```python
from build123d import *

# Parameters (mm, degrees)
F0_R      = 56.35625
F1_DEPTH  = 2120.9
F2_R      = 50.8
F3_DEPTH  = 368.3
F4_R      = 11.1125
F5_DEPTH  = 34.925
F6_W      = 25.4
F6_H      = 25.4
F7_DEPTH  = 355.6
F8_R      = 12.699
F11_DEPTH = 13.97


# Not quite as in the source:
# - a fillet or chamfer is up to 0.001 mm smaller than in the source, because OpenCascade refuses the exact size


with BuildPart() as f1:
    # F0 (on Front) → F1 (new body)
    with BuildSketch(Plane.XZ):
        Circle(F0_R)
    extrude(amount=-F1_DEPTH)

    # F2 (on face) → F3 (join)
    with BuildSketch(Plane(origin=(0, 2120.9, 0), x_dir=(-1, 0, 0), z_dir=(0, 1, 0))):
        Circle(F2_R)
    extrude(amount=F3_DEPTH)

    # F4 (on face) → F5 (cut)
    with BuildSketch(Plane(origin=(0, 2489.2, 0), x_dir=(-1, 0, 0), z_dir=(0, 1, 0))):
        Circle(F4_R)
    extrude(amount=-F5_DEPTH, mode=Mode.SUBTRACT)

    # F6 (on face) → F7 (cut)
    with BuildSketch(Plane(origin=(0, 2489.2, 0), x_dir=(-1, 0, 0), z_dir=(0, 1, 0))):
        with Locations((0, 49.53)):
            Rectangle(F6_W, F6_H)
    extrude(amount=-F7_DEPTH, mode=Mode.SUBTRACT)

    # F8 (radius 12.7 in the source; OpenCascade refuses exactly that, so slightly less here)
    f8_edges = [f1.edges().sort_by_distance(p)[0] for p in [
        (12.7, 2133.6, 43.008444),
        (-12.7, 2133.6, 43.008444),
    ]]
    fillet(f8_edges, radius=F8_R)

    # F10 (on offset) → F11 (cut)
    with BuildSketch(Plane.XY.offset(56.35625)):
        with BuildLine():
            ThreePointArc((0, 477.8375), (-8.9802561211, 474.1177561211), (-12.7, 465.1375))
            Line((-12.7, 465.1375), (-12.7, 287.3375))
            ThreePointArc((-12.7, 287.3375), (-8.9802561211, 278.3572438789), (0, 274.6375))
            ThreePointArc((0, 274.6375), (8.9802561211, 278.3572438789), (12.7, 287.3375))
            Line((12.7, 287.3375), (12.7, 465.1375))
            ThreePointArc((12.7, 465.1375), (8.9802561211, 474.1177561211), (0, 477.8375))
        make_face()
        with BuildLine():
            ThreePointArc((0, 1782.7625), (-8.9802561211, 1779.0427561211), (-12.7, 1770.0625))
            Line((-12.7, 1770.0625), (-12.7, 1592.2625))
            ThreePointArc((-12.7, 1592.2625), (-8.9802561211, 1583.2822438789), (0, 1579.5625))
            ThreePointArc((0, 1579.5625), (8.9802561211, 1583.2822438789), (12.7, 1592.2625))
            Line((12.7, 1592.2625), (12.7, 1770.0625))
            ThreePointArc((12.7, 1770.0625), (8.9802561211, 1779.0427561211), (0, 1782.7625))
        make_face()
    extrude(amount=-F11_DEPTH, mode=Mode.SUBTRACT)


solid = f1.part
```
The model under review builds one solid part; all positions refer to its coordinate system, in mm. A direction names the side the tool comes from. Coordinates: 2 decimals unless noted, no trailing zeros. Write each loop counter-clockwise with the first axis right and the second up, starting at its lowest first coordinate (ties: lowest second). Pieces come first, ordered by that corner, then holes. Notation, with made-up numbers: (86, 39) -> (90, 39) arc R11 ccw to (90, 58) -> close; hole circle Ø5 at (51.5, 81.5). An arc over 180 degrees is marked (long way). One line per item, written item: value. Start each with the question number.
Q1. Add section C-C, the plane y = 2200. Give the boundary of the cut face in (x, z), then the cut area to 3 significant figures.
Q2. Add section A-A, the plane y = 1328. Give the boundary of the cut face in (x, z).
Q3. Clearance check with flat-ended pins moving along their axes: P1, Ø2, axis at y = 1977, z = -30.5, coming from the -X side; P2, Ø4, axis at x = -34, y = 1363, coming from the +Z side; P3, Ø14, axis at y = 1680.5, z = 47, coming from the -X side; P4, Ø12, axis at x = 3, z = -6, coming from the -Y side. State where each tip first meets the part, or that it passes through.
Q4. Add section B-B, the plane y = 1627.5. Give the boundary of the cut face in (x, z).
Q5. For faces 1 (the face through (-8.6, 2120.9, 50.4)), 2 (the face through (-12.217, 1045.604, -55.016)), list the 3-axis set-ups (+Z, -Z, +X, -X, +Y, -Y) from which the entire face can be reached by the end or side of a thin tool; tool diameter is ignored.
Q6. To check wall thickness, follow probe 1 along Z at (x, y) = (0, 2479); probe 2 along X at (y, z) = (2188.5, -4); probe 3 along X at (y, z) = (1135.5, -7). State the ranges of each line that lie inside material, in increasing order.
Response:
1. outline: (-12.7, 36.83) -> (-12.7, 49.19) arc R50.8 ccw (long way) to (12.7, 49.19) -> (12.7, 36.83) -> close
1. area: 7,770 mm²
2. outline: circle Ø112.71 at (0, 0)
3. P1: x = -48.02
3. P2: z = 46.39
3. P3: x = -39.7
3. P4: y = 0
4. outline: (-12.7, 42.39) -> (-12.7, 54.91) arc R56.36 ccw (long way) to (12.7, 54.91) -> (12.7, 42.39) -> close
5. face 1: +Y
5. face 2: +Y, -Y
6. probe 1: -50.8 to -11.11, 11.11 to 36.83
6. probe 2: -50.64 to 50.64
6. probe 3: -55.92 to 55.92
